```python
from build123d import *

# Parameters (mm, degrees)
BOSS_EXTRUDE1_DEPTH      = 101.6
BOSS_EXTRUDE2_REACH      = 145.704
BOSS_EXTRUDE2_END_RADIUS = 180.975
BOSS_EXTRUDE3_REACH      = 145.807
BOSS_EXTRUDE3_END_RADIUS = 180.975


with BuildPart() as part:
    # Sketch1 → Boss-Extrude1 (new body)
    with BuildSketch(Plane.XY):
        with BuildLine():
            Line((0, 79.375), (0, 180.975))
            ThreePointArc((0, 180.975), (1.579284762, 180.968109027), (3.158449255, 180.947436631))
            Line((3.158449255, 180.947436631), (1.385284761, 79.362910803))
            ThreePointArc((1.385284761, 79.362910803), (0.692668755, 79.371977643), (0, 79.375))
        make_face()
    extrude(amount=BOSS_EXTRUDE1_DEPTH)

    # Boss-Extrude2: up to this cylinder (the profile starts inside it)
    boss_extrude2_end = Plane(origin=(0, 0, 50.8), z_dir=(0, 0, -1)) * Cylinder(BOSS_EXTRUDE2_END_RADIUS, 730.558, mode=Mode.PRIVATE)
    # Sketch2 → Boss-Extrude2 (add, up to the surface)
    with BuildSketch(Plane(origin=(1.385284761, 79.362910803, 0), x_dir=(0, 0, -1), z_dir=(-0.017452406437283553, -0.9998476951563913, 0)), mode=Mode.PRIVATE) as boss_extrude2_sk1:
        Polygon((-92.000208065, 0), (-93.4085, 2.794), (-84.3915, 2.794), (-85.799791935, 0), align=None)
    boss_extrude2_tool1 = extrude(boss_extrude2_sk1.sketch, amount=-BOSS_EXTRUDE2_REACH, mode=Mode.PRIVATE) & boss_extrude2_end
    add(boss_extrude2_tool1.solids().sort_by_distance((2.868249, 79.337026, 88.9))[0])
    # Sketch2 → Boss-Extrude2 (add, up to the surface)
    with BuildSketch(Plane(origin=(1.385284761, 79.362910803, 0), x_dir=(0, 0, -1), z_dir=(-0.017452406437283553, -0.9998476951563913, 0)), mode=Mode.PRIVATE) as boss_extrude2_sk2:
        Polygon((-15.800208065, 0), (-9.599791935, 0), (-8.1915, 2.794), (-17.2085, 2.794), align=None)
    boss_extrude2_tool2 = extrude(boss_extrude2_sk2.sketch, amount=-BOSS_EXTRUDE2_REACH, mode=Mode.PRIVATE) & boss_extrude2_end
    add(boss_extrude2_tool2.solids().sort_by_distance((2.868249, 79.337026, 12.7))[0])

    # Boss-Extrude3: up to this cylinder (the profile starts inside it)
    boss_extrude3_end = Plane(origin=(0, 0, 50.8), z_dir=(0, 0, -1)) * Cylinder(BOSS_EXTRUDE3_END_RADIUS, 730.764, mode=Mode.PRIVATE)
    # Sketch3 → Boss-Extrude3 (add, up to the surface)
    with BuildSketch(Plane(origin=(0, 79.375, 0), x_dir=(0, 0, -1), z_dir=(0, -1, 0)), mode=Mode.PRIVATE) as boss_extrude3_sk1:
        Polygon((-92.000208065, 0), (-93.4085, -2.79357446), (-84.3915, -2.79357446), (-85.799791935, 0), align=None)
    boss_extrude3_tool1 = extrude(boss_extrude3_sk1.sketch, amount=-BOSS_EXTRUDE3_REACH, mode=Mode.PRIVATE) & boss_extrude3_end
    add(boss_extrude3_tool1.solids().sort_by_distance((-1.482964, 79.375, 88.9))[0])
    # Sketch3 → Boss-Extrude3 (add, up to the surface)
    with BuildSketch(Plane(origin=(0, 79.375, 0), x_dir=(0, 0, -1), z_dir=(0, -1, 0)), mode=Mode.PRIVATE) as boss_extrude3_sk2:
        Polygon((-15.800208065, 0), (-9.599791935, 0), (-8.1915, -2.79357446), (-17.2085, -2.79357446), align=None)
    boss_extrude3_tool2 = extrude(boss_extrude3_sk2.sketch, amount=-BOSS_EXTRUDE3_REACH, mode=Mode.PRIVATE) & boss_extrude3_end
    add(boss_extrude3_tool2.solids().sort_by_distance((-1.482964, 79.375, 12.7))[0])


solid = part.part
```
Verification items for the finished model (mm, model axes). Coordinates: 2 decimals unless noted, no trailing zeros. Loops run counter-clockwise (first coordinate to the right, second up) from the corner with the lowest first, then second, coordinate; pieces in that order, holes last. Notation, with made-up numbers: (52.25, 47) - (72.25, 47) arc R29 cw to (72.25, 75) - close; hole circle Ø2 at (8.25, 4.5). An arc over 180 degrees is marked (long way). Put each result on its own line as item: value.
Item 1: Section check B-B (z = 34.5). Enter the section's corners in (x, y) (3 decimals).
Conclusion:
outline: (0, 79.375) arc R79.375 cw to (1.385, 79.363) - (3.158, 180.947) arc R180.975 ccw to (0, 180.975) - close
Item 2: Section check A-A (y = 154.5). Enter the section's corners in (x, z), then the cut area to 3 significant figures.
Conclusion:
outline: (-2.79, 8.19) - (0, 9.6) - (0, 0) - (2.7, 0) - (2.7, 9.6) - (5.49, 8.19) - (5.49, 17.21) - (2.7, 15.8) - (2.7, 85.8) - (5.49, 84.39) - (5.49, 93.41) - (2.7, 92) - (2.7, 101.6) - (0, 101.6) - (0, 92) - (-2.79, 93.41) - (-2.79, 84.39) - (0, 85.8) - (0, 15.8) - (-2.79, 17.21) - close
area: 359 mm2
Item 3: Section check C-C (y = 97.5). Enter the section's corners in (x, z), then the cut area to 3 significant figures.
Conclusion:
outline: (-2.79, 8.19) - (0, 9.6) - (0, 0) - (1.7, 0) - (1.7, 9.6) - (4.5, 8.19) - (4.5, 17.21) - (1.7, 15.8) - (1.7, 85.8) - (4.5, 84.39) - (4.5, 93.41) - (1.7, 92) - (1.7, 101.6) - (0, 101.6) - (0, 92) - (-2.79, 93.41) - (-2.79, 84.39) - (0, 85.8) - (0, 15.8) - (-2.79, 17.21) - close
area: 258 mm2
Item 4: Scan lines: line 1 along X through (y, z) = (96.5, 17); line 2 along Z through (x, y) = (3.5, 144); line 3 along Y through (x, z) = (1.5, 88.5). Record each from-to range of solid material in increasing order.
Conclusion:
line 1: x = -2.79 to -2.38, 0 to 1.68, 4.07 to 4.48
line 2: z = 9.1 to 16.3, 85.3 to 92.5
line 3: y = 79.36 to 180.97
Item 5: Gauge pin test, flat ends, axial feed: pin 1 Ø3 at (y, z) = (126.5, 95) entering from -X; pin 2 Ø3 at (x, z) = (-1.5, 87) entering from -Y (3 decimals); pin 3 Ø1.5 at (y, z) = (165, 52) entering from +X. Record the tip position at first contact, or that the pin passes through.
Conclusion:
pin 1: stops at x = 0
pin 2: stops at y = 79.375
pin 3: stops at x = 2.89
Item 6: Draft check along X on faces 1 (the face through (-1.416, 129.464, 16.514)), 2 (the face through (-1.377, 129.464, 92.694)), 3 (the face through (1, 142, 101.6)), 4 (the face through (-2.794, 129, 89)). Enter one of: pulls with the +X half, pulls with the -X half, needs draft (parallel to the pull), parting line crosses it, or undercut.
Conclusion:
face 1: undercut
face 2: undercut
face 3: needs draft
face 4: pulls with the -X half
